```python
from build123d import *

# Parameters (mm, degrees)
PAD_DEPTH = 7
FILLET_R  = 1


with BuildPart() as part:
    # Sketch → Pad (new body)
    with BuildSketch(Plane.XY):
        with BuildLine():
            Line((-10, 20), (10, 20))
            Line((10, 20), (10, 0))
            ThreePointArc((-10, 0), (0, -10), (10, 0))
            Line((-10, 0), (-10, 20))
        make_face()
    extrude(amount=PAD_DEPTH)

    # Fillet
    fillet_edges = [part.edges().sort_by_distance(p)[0] for p in [
        (-10, 20, 3.5),
        (10, 20, 3.5),
    ]]
    fillet(fillet_edges, radius=FILLET_R)


solid = part.part
```
The model under review builds one solid part; all positions refer to its coordinate system, in mm. Round coordinates to 2 decimals unless told otherwise and drop trailing zeros. Loops run counter-clockwise (first coordinate to the right, second up) from the corner with the lowest first, then second, coordinate; pieces in that order, holes last. Notation, with made-up numbers: M 65,-7.75 L 124,-7.75 A21 cw 124,0.25 Z; hole C 39,27 d11. An arc over 180 degrees is marked long. Answer as a JSON object with one key per item and string values.
(1) Take a section at A-A on x = -8. Give the boundary of the cut face in (y, z).
Resolved:
{"outline": "M -6,0 L 20,0 L 20,7 L -6,7 Z"}
(2) Take a section at B-B on z = 3. Give the boundary of the cut face in (x, y).
Resolved:
{"outline": "M -10,0 A10 ccw 10,0 L 10,19 A1 ccw 9,20 L -9,20 A1 ccw -10,19 Z"}
(3) To check wall thickness, follow line 1 along Y through (x, z) = (0.25, 6.5); line 2 along Y through (x, z) = (7.5, 0.75); line 3 along X through (y, z) = (-6.75, 5). State the ranges of each line that lie inside material, in increasing order.
Resolved:
{"line 1": "-10 to 20", "line 2": "-6.61 to 20", "line 3": "-7.38 to 7.38"}
(4) Take a section at C-C on y = -5.25. Give the boundary of the cut face in (x, z).
Resolved:
{"outline": "M -8.51,0 L 8.51,0 L 8.51,7 L -8.51,7 Z"}
(5) Draft analysis for pull direction Z (two halves, no side actions). For faces 1 (the flat face through (0, 5, 0)), 2 (the cylindrical face through (-9.699, 19.715, 3.549)), 3 (the flat face through (0, 5, 7)), state which applies: released by +Z, released by -Z, zero draft, split by the parting line, or undercut.
Resolved:
{"face 1": "released by -Z", "face 2": "zero draft", "face 3": "released by +Z"}
